from build123d import *

# Parameters (mm, degrees)
SKETCH_1_W          = 20
SKETCH_1_H          = 60
EXTRUDE_1_DEPTH     = 3
SKETCH_2_W          = 60
SKETCH_2_H          = 20
EXTRUDE_2_DEPTH     = 3
SKETCH_3_R          = 2
CUT_EXTRUDE_1_DEPTH = 3
FILLET_3_R          = 5
FILLET_2_R          = 3


with BuildPart() as part:
    # 草图1 → 凸台-拉伸1 (new body)
    with BuildSketch(Plane.XY):
        with Locations((10, 30)):
            Rectangle(SKETCH_1_W, SKETCH_1_H)
    extrude(amount=EXTRUDE_1_DEPTH)

    # 草图2 → 凸台-拉伸2 (add)
    with BuildSketch(Plane.XY.offset(3)):
        with Locations((-10, 10)):
            Rectangle(SKETCH_2_W, SKETCH_2_H)
    extrude(amount=-EXTRUDE_2_DEPTH)

    # 草图3 → 切除-拉伸1 (cut)
    with BuildSketch(Plane.XY.offset(3)):
        with Locations((10, 10)):
            Circle(SKETCH_3_R)
        with Locations((10, 30)):
            Circle(SKETCH_3_R)
        with Locations((10, 50)):
            Circle(SKETCH_3_R)
        with Locations(Location((-10, 10, 0), (0, 0, 180))):
            Circle(SKETCH_3_R)
        with Locations(Location((-30, 10, 0), (0, 0, 180))):
            Circle(SKETCH_3_R)
    extrude(amount=-CUT_EXTRUDE_1_DEPTH, mode=Mode.SUBTRACT)

    # 圆角3
    fillet_3_edges = [part.edges().sort_by_distance(p)[0] for p in [
        (0, 20, 1.5),
        (20, 0, 1.5),
    ]]
    fillet(fillet_3_edges, radius=FILLET_3_R)

    # 圆角2
    fillet_2_edges = [part.edges().sort_by_distance(p)[0] for p in [
        (-40, 20, 1.5),
        (-40, 0, 1.5),
        (0, 60, 1.5),
        (20, 60, 1.5),
    ]]
    fillet(fillet_2_edges, radius=FILLET_2_R)


solid = part.part
Verification items for the finished model (mm, model axes). A direction names the side the tool comes from. Round coordinates to 2 decimals unless told otherwise and drop trailing zeros. Order: outer loops, then holes, each group sorted by start corner. A loop starts at its lowest first (then second) coordinate and runs counter-clockwise, first axis right, second up.
1. Release check for a two-part mould opening along X. For faces 3 (the cylindrical face through (10, 28, 2)), 4 (the cylindrical face through (18, 1, 2)), 5 (the flat face through (-40, 10, 2)) record: +X half, -X half, draft (parallel to the pull), parting line (faces both ways), or undercut.
Final values:
face 3: undercut
face 4: +X half
face 5: -X half
2. Access from +Z, -Z, +X, -X, +Y, -Y to the whole of each face (thin tool, end or side, straight path). Record for faces 1 (the flat face through (0, 41, 1)), 2 (the flat face through (3, 24, 0)).
Final values:
face 1: +Z, -Z, -X, +Y
face 2: -Z, +X, -X, +Y, -Y
3. Section check A-A on y = 30. Record the cut outline in (x, z).
Final values:
outline: (0, 0) - (8, 0) - (8, 3) - (0, 3) - close; (12, 0) - (20, 0) - (20, 3) - (12, 3) - close
4. Section check C-C on z = 2.35. Record the cut outline in (x, y).
Final values:
outline: (-40, 3) arc R3 ccw to (-37, 0) - (15, 0) arc R5 ccw to (20, 5) - (20, 57) arc R3 ccw to (17, 60) - (3, 60) arc R3 ccw to (0, 57) - (0, 25) arc R5 cw to (-5, 20) - (-37, 20) arc R3 ccw to (-40, 17) - close; hole circle Ø4 at (-30, 10); hole circle Ø4 at (-10, 10); hole circle Ø4 at (10, 10); hole circle Ø4 at (10, 30); hole circle Ø4 at (10, 50)
5. Section check D-D on y = 10. Record the cut outline in (x, z).
Final values:
outline: (-40, 0) - (-32, 0) - (-32, 3) - (-40, 3) - close; (-28, 0) - (-12, 0) - (-12, 3) - (-28, 3) - close; (-8, 0) - (8, 0) - (8, 3) - (-8, 3) - close; (12, 0) - (20, 0) - (20, 3) - (12, 3) - close
6. Section check B-B on x = 10. Record the cut outline in (y, z), then the cut area to 3 significant figures.
Final values:
outline: (0, 0) - (8, 0) - (8, 3) - (0, 3) - close; (12, 0) - (28, 0) - (28, 3) - (12, 3) - close; (32, 0) - (48, 0) - (48, 3) - (32, 3) - close; (52, 0) - (60, 0) - (60, 3) - (52, 3) - close
area: 144 mm2
7. Thickness scan on L1, parallel to Y at x = 10, z = 1.3; L2, parallel to Y at x = -30, z = 1.15; L3, parallel to X at y = 9.5, z = 1.95. Record the ranges inside material, lowest first.
Final values:
L1: y = 0 to 8, 12 to 28, 32 to 48, 52 to 60
L2: y = 0 to 8, 12 to 20
L3: x = -40 to -31.94, -28.06 to -11.94, -8.06 to 8.06, 11.94 to 20
